Geometry: final body of the model. Coordinates: model frame, mm. Face numbers are marked on the shaded views. Round coordinates to 2 decimals unless told otherwise and drop trailing zeros. Write each loop counter-clockwise with the first axis right and the second up, starting at its lowest first coordinate (ties: lowest second). Pieces come first, ordered by that corner, then holes. Notation, with made-up numbers: (72.25, 6) -> (84.25, 6) arc R15 ccw to (84.25, 23) -> close; hole circle Ø7 at (85, 52). An arc over 180 degrees is marked (long way). Use one line per item in the form item = value. Start each with the question number.
1. Draft query along Z for the marked faces 1, 2, 3 and 4. Return one class per face: pulls with the +Z half, pulls with the -Z half, needs draft (parallel to the pull), parting line crosses it, or undercut.
2. Cut plane A-A, the plane x = 0. Return the cut outline in (y, z), plus the area to 3 significant figures.
3. Cut plane B-B, the plane y = 0. Return the cut outline in (x, z), plus the area to 3 significant figures.
4. Line query: L1, parallel to X at y = -2.5, z = -1.5; L2, parallel to Z at x = -1.5, y = 2.5; L3, parallel to X at y = 1.25, z = -3.25. Output: solid intervals per line, ascending.
5. Pin query (flat end, axial travel): pin 1 Ø5 at (x, y) = (3.5, -3.5) entering from +Z; pin 2 Ø2 at (y, z) = (-1, 2) entering from -X. Return the tip coordinate at first contact, or that it passes through.
6. Cut plane C-C, the plane y = 3. Return the cut outline in (x, z).
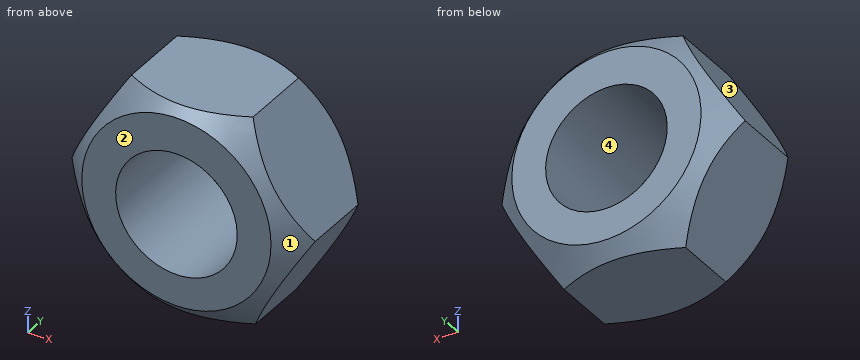
```python
from build123d import *

# Parameters (mm, degrees)
SKETCH1_R           = 4.5
BOSS_EXTRUDE1_DEPTH = 4.5
SKETCH2_OUTSIDE_W   = 43.092
SKETCH2_OUTSIDE_H   = 40.68
SKETCH2_OUTSIDE_R   = 7
CUT_EXTRUDE2_DEPTH  = 9
CUT_EXTRUDE2_TAPER  = 45


with BuildPart() as part:
    # Sketch1 → Boss-Extrude1 (new body, symmetric)
    with BuildSketch(Plane(origin=(0, 0, 0), x_dir=(1, 0, 0), z_dir=(0, 1, 0))):
        Polygon((-4.5, -7.794228634), (4.5, -7.794228634), (9, 0), (4.5, 7.794228634), (-4.5, 7.794228634), (-9, 0), align=None)
        with Locations(Location((0, 0, 0), (0, 0, 270))):  # turned: the seam where the file's is
            Circle(SKETCH1_R, mode=Mode.SUBTRACT)
    extrude(amount=BOSS_EXTRUDE1_DEPTH, both=True)

    # Sketch2 outside → Cut-Extrude2 (cut)
    with BuildSketch(Plane(origin=(0, 4.5, 0), x_dir=(1, 0, 0), z_dir=(0, 1, 0))):
        Rectangle(SKETCH2_OUTSIDE_W, SKETCH2_OUTSIDE_H)
        with Locations((0, -0.176410187)):
            Circle(SKETCH2_OUTSIDE_R, mode=Mode.SUBTRACT)
    cut_extrude2 = extrude(amount=-CUT_EXTRUDE2_DEPTH, taper=CUT_EXTRUDE2_TAPER, mode=Mode.SUBTRACT)

    # Mirror4: Cut-Extrude2 across plane
    add(cut_extrude2.mirror(Plane.ZX), mode=Mode.SUBTRACT)


solid = part.part
```
Outcome:
q1.face_1 = parting line crosses it
q1.face_2 = needs draft
q1.face_3 = pulls with the +Z half
q1.face_4 = undercut
q2.outline = (-4.5, -6.82) -> (-3.53, -7.79) -> (3.53, -7.79) -> (4.5, -6.82) -> (4.5, -4.5) -> (-4.5, -4.5) -> close; (-4.5, 4.5) -> (4.5, 4.5) -> (4.5, 7.18) -> (3.88, 7.79) -> (-3.88, 7.79) -> (-4.5, 7.18) -> close
q2.area = 58.0 mm^2
q3.outline = (-9, 0) -> (-4.5, -7.79) -> (4.5, -7.79) -> (9, 0) -> (4.5, 7.79) -> (-4.5, 7.79) -> close; hole circle Ø9 at (0, 0)
q3.area = 147 mm^2
q4.L1 = -8.13 to -4.24, 4.24 to 8.13
q4.L2 = -7.79 to -4.24, 4.24 to 7.79
q4.L3 = -7.12 to -3.11, 3.11 to 7.12
q5.pin_1 = 7.79
q5.pin_2 = -8.42
q6.outline = (-8.47, 0.92) arc R8.5 ccw to (-8.42, -1.01) -> (-5.24, -6.52) arc R8.5 ccw to (-2.95, -7.79) -> (2.95, -7.79) arc R8.5 ccw to (5.24, -6.52) -> (8.42, -1.01) arc R8.5 ccw to (8.47, 0.92) -> (4.88, 7.14) arc R8.5 ccw to (3.77, 7.79) -> (-3.77, 7.79) arc R8.5 ccw to (-4.88, 7.14) -> close; hole circle Ø9 at (0, 0)
